Can you work these out from the model? Positions are in its coordinate system, mm. Face numbers are marked on the shaded views. A direction names the side the tool comes from. Give positions to 0.01 mm unless a question says otherwise; leave off trailing zeros. Write each loop counter-clockwise with the first axis right and the second up, starting at its lowest first coordinate (ties: lowest second). Pieces come first, ordered by that corner, then holes. Notation, with made-up numbers: (-35.75, -27.5) -> (7.25, -27.5) arc R24 cw to (7.25, 10.5) -> close; hole circle Ø4 at (-23, 67). An arc over 180 degrees is marked (long way). Answer as CSV lines item,"result". Start each with the question number.
1. On a 3-axis mill with a long thin cutter (end or side, diameter ignored), from which of +Z, -Z, +X, -X, +Y, -Y can I reach the whole of each face in a straight line? I mean the marked faces 3 and 4. Say none if no direction works.
2. If we mould it in two halves opening along Z, with no side actions, what happens to the marked faces 1 and 2? For each: pulls with the +Z half, pulls with the -Z half, needs draft (parallel to the pull), parting line crosses it, or undercut.
3. If we section it at A-A on y = -10.25: Write out the boundary of the cut face in (x, z) (3 decimals), plus the area to 3 significant figures.
4. I need wall thicknesses on line 1 (Z direction, x = -11, y = 2.5); line 2 (Z direction, x = 3.5, y = 0); line 3 (X direction, y = -1, z = -25.5) (3 decimals). Which ranges of each line are inside material? Lowest first, please. Write a range as [from, to].
5. I'm going to push flat-ended pins straight in: P1, Ø6.5, axis at y = -1, z = 12.5, coming from the +X side; P2, Ø0.8, axis at y = 1, z = 2, coming from the +X side; P3, Ø0.8, axis at y = -1, z = -2, coming from the -X side. Where does each tip first touch, or does it pass through?
6. If we section it at B-B on z = -26.5: Count the separate pieces of the cut face and the enclosed holes in it, plus the area to 3 significant figures.
```python
from build123d import *

# Parameters (mm, degrees)
F1_DEPTH = 3
F2_COUNT = 6
F3_R     = 35.35
F4_DEPTH = 9.5
F5_R     = 7
F6_R     = 3.5
F7_DEPTH = 3
F8_W     = 1.55
F8_H     = 1.8
F8_W_2   = 1.8
F8_H_2   = 1.55
F9_DEPTH = 25
F10_R    = 0.5


with BuildPart() as f1:
    # F0 (on Front) → F1 (new body, symmetric)
    with BuildSketch(Plane.XZ):
        with BuildLine():
            ThreePointArc((-2.775, 2.1329263935), (-4.6419e-05, 3.4999999997), (2.7749434229, 2.133))
            Line((2.7749434229, 2.133), (2.7749434229, 27.7114090042))
            ThreePointArc((2.7749434229, 27.7114090042), (1.3891728178, 27.8153320829), (-5.65771e-05, 27.8499999999))
            ThreePointArc((-5.65771e-05, 27.8499999999), (-1.3892577191, 27.8153278426), (-2.775, 27.7114033387))
            Line((-2.775, 27.7114033387), (-2.775, 2.1329263935))
        make_face()
    extrude(amount=F1_DEPTH, both=True)

    # F2: F1 ×6 about axis
    f2_axis = Axis((0, 0, 0), (0, -1, 0))


with BuildPart() as f1_1:
    add(f1.part)
    for i in range(1, F2_COUNT):
        add(f1.part.rotate(f2_axis, i * 360 / F2_COUNT))

    # F3 (on face) → F4 (join, symmetric)
    with BuildSketch(Plane.XZ.offset(3)):
        Circle(F3_R)
        with BuildLine():
            ThreePointArc((25.3862558838, 11.4525330038), (27.2270979574, 5.8572721312), (27.85, 0))
            ThreePointArc((27.85, 0), (27.2271039366, -5.857244337), (25.3862792658, -11.4524811738))
            ThreePointArc((25.3862792658, -11.4524811738), (24.7834093858, -12.7045314441), (24.1188357839, -13.9249510028))
            ThreePointArc((24.1188357839, -13.9249510028), (23.3941977896, -15.1107249919), (22.6113124609, -16.2588760004))
            ThreePointArc((22.6113124609, -16.2588760004), (13.9250246211, -24.1187932804), (2.775, -27.7114033387))
            ThreePointArc((2.775, -27.7114033387), (1.3892577191, -27.8153278426), (5.65771e-05, -27.8499999999))
            ThreePointArc((5.65771e-05, -27.8499999999), (-1.3891728178, -27.8153320829), (-2.7749434229, -27.7114090042))
            ThreePointArc((-2.7749434229, -27.7114090042), (-13.9249753789, -24.1188217104), (-22.6112792658, -16.2589221649))
            ThreePointArc((-22.6112792658, -16.2589221649), (-23.3941516667, -15.1107963985), (-24.1187792068, -13.9250489972))
            ThreePointArc((-24.1187792068, -13.9250489972), (-24.7833706074, -12.704607091), (-25.3862558838, -11.4525330038))
            ThreePointArc((-25.3862558838, -11.4525330038), (-27.85, -2.843e-05), (-25.3862792658, 11.4524811738))
            ThreePointArc((-25.3862792658, 11.4524811738), (-24.7834093858, 12.7045314441), (-24.1188357839, 13.9249510028))
            ThreePointArc((-24.1188357839, 13.9249510028), (-23.3941977896, 15.1107249919), (-22.6113124609, 16.2588760004))
            ThreePointArc((-22.6113124609, 16.2588760004), (-13.9250246211, 24.1187932804), (-2.775, 27.7114033387))
            ThreePointArc((-2.775, 27.7114033387), (-1.3892577191, 27.8153278426), (-5.65771e-05, 27.8499999999))
            ThreePointArc((-5.65771e-05, 27.8499999999), (1.3891728178, 27.8153320829), (2.7749434229, 27.7114090042))
            ThreePointArc((2.7749434229, 27.7114090042), (13.9249753789, 24.1188217104), (22.6112792658, 16.2589221649))
            ThreePointArc((22.6112792658, 16.2589221649), (23.3941516667, 15.1107963985), (24.1187792068, 13.9250489972))
            ThreePointArc((24.1187792068, 13.9250489972), (24.7833706074, 12.704607091), (25.3862558838, 11.4525330038))
        make_face(mode=Mode.SUBTRACT)
    extrude(amount=F4_DEPTH, both=True)

    # F5
    f5_edges = [f1_1.edges().sort_by_distance(p)[0] for p in [
        (-35.35, 6.5, 0),
        (-35.35, -12.5, 0),
    ]]
    fillet(f5_edges, radius=F5_R)

    # F6 (on Front) → F7 (join, symmetric)
    with BuildSketch(Plane.XZ):
        Circle(F6_R)
    extrude(amount=F7_DEPTH, both=True)

    # F8 (on face) → F9 (cut)
    with BuildSketch(Plane.XZ.offset(3)):
        with Locations((-1.675, 0)):
            Rectangle(F8_W, F8_H)
        with Locations((0, 1.675)):
            Rectangle(F8_W_2, F8_H_2)
        Rectangle(F8_W_2, F8_H)
        with Locations((1.675, 0)):
            Rectangle(F8_W, F8_H)
        with Locations((0, -1.675)):
            Rectangle(F8_W_2, F8_H_2)
    extrude(amount=-F9_DEPTH, mode=Mode.SUBTRACT)

    # F10
    f10_edges = [f1_1.edges().sort_by_distance(p)[0] for p in [
        (0.9, 0, 0.9),
        (0.9, 0, -0.9),
        (-0.9, 0, -0.9),
        (-0.9, 0, 0.9),
    ]]
    fillet(f10_edges, radius=F10_R)


solid = f1_1.part
```
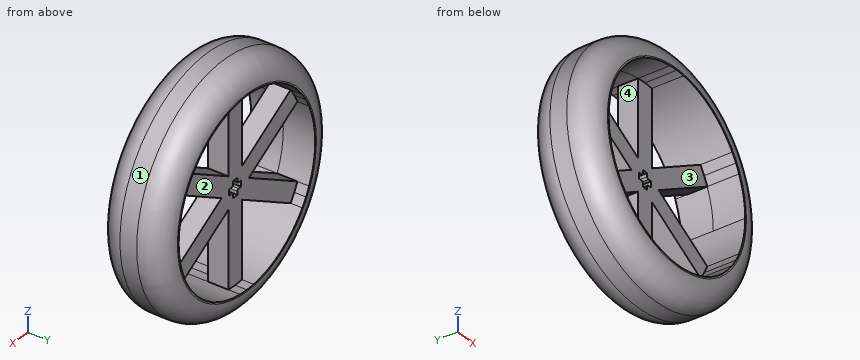
Computed values:
1,face 3,"-Y"
1,face 4,"+Y, -Y"
2,face 1,"parting line crosses it"
2,face 2,"undercut"
3,outline,"circle Ø66.983 at (0, 0); hole circle Ø55.7 at (0, 0)"
3,area,"1,090 mm2"
4,line 1,"z = [-32.88, -25.59], [-9.56, -3.15], [3.15, 9.56], [25.59, 32.88]"
4,line 2,"z = [-35.16, -27.63], [-5.22, 5.23], [27.63, 35.16]"
4,line 3,"x = [-24.482, -11.197], [-2.775, 2.775], [11.197, 24.482]"
5,P1,"stops at x = 34.12"
5,P2,"stops at x = 35.21"
5,P3,"stops at x = -35.31"
6,separate pieces,"3"
6,enclosed holes,"0"
6,area,"528 mm2"
